Could you check a few things on this model? Use its own coordinates, in mm. A direction names the side the tool comes from. Round coordinates to 2 decimals unless told otherwise and drop trailing zeros. One line per question, with ' | ' between items.
```python
from build123d import *

# Parameters (mm, degrees)
F0_W      = 101.6
F0_H      = 25.4
F1_DEPTH  = 101.6
F1_FACE_W = 101.6
F1_FACE_H = 101.6
F6_DEPTH  = 50.8
F8_DEPTH  = 63.5


with BuildPart() as f1:
    # F0 (on Front) → F1 (new body)
    with BuildSketch(Plane.XZ):
        with Locations((-50.8, -12.7)):
            Rectangle(F0_W, F0_H)
    extrude(amount=F1_DEPTH)

    # F1_face (on face) → F4 section 0
    with BuildSketch(Plane(origin=(-50.8, -50.8, 0), x_dir=(1, 0, 0), z_dir=(0, 0, 1))):
        Rectangle(F1_FACE_W, F1_FACE_H)
    # F3 (on offset) → F4 section 1
    with BuildSketch(Plane.XY.offset(323.85)):
        Polygon((0, -50.8), (-50.8, 0), (-101.6, -50.8), (-50.8, -101.6), align=None)
    loft()

    # F5 (on face) → F6 (cut)
    with BuildSketch(Plane.XY.offset(323.85)):
        with BuildLine():
            ThreePointArc((-46.3098719395, -46.3098719395), (-50.8, -44.45), (-55.2901280605, -46.3098719395))
            Line((-55.2901280605, -46.3098719395), (-50.8, -50.8))
            Line((-50.8, -50.8), (-46.3098719395, -46.3098719395))
        make_face()
        with BuildLine():
            Line((-50.8, -50.8), (-55.2901280605, -46.3098719395))
            ThreePointArc((-55.2901280605, -46.3098719395), (-57.15, -50.8), (-55.2901280605, -55.2901280605))
            Line((-55.2901280605, -55.2901280605), (-50.8, -50.8))
        make_face()
        with BuildLine():
            Line((-46.3098719395, -55.2901280605), (-50.8, -50.8))
            Line((-50.8, -50.8), (-55.2901280605, -55.2901280605))
            ThreePointArc((-55.2901280605, -55.2901280605), (-50.8, -57.15), (-46.3098719395, -55.2901280605))
        make_face()
        with BuildLine():
            Line((-46.3098719395, -46.3098719395), (-50.8, -50.8))
            Line((-50.8, -50.8), (-46.3098719395, -55.2901280605))
            ThreePointArc((-46.3098719395, -55.2901280605), (-44.9333649686, -53.2300397955), (-44.45, -50.8))
            ThreePointArc((-44.45, -50.8), (-44.9333649686, -48.3699602045), (-46.3098719395, -46.3098719395))
        make_face()
    extrude(amount=-F6_DEPTH, mode=Mode.SUBTRACT)

    # F7 (on face) → F8 (cut)
    with BuildSketch(Plane(origin=(0, 0, -25.4), x_dir=(1, 0, 0), z_dir=(0, 0, -1))):
        with BuildLine():
            ThreePointArc((-41.275, 50.8), (-44.0648079092, 57.5351920908), (-50.8, 60.325))
            Line((-50.8, 60.325), (-50.8, 41.275))
            ThreePointArc((-50.8, 41.275), (-44.0648079092, 44.0648079092), (-41.275, 50.8))
        make_face()
        with BuildLine():
            Line((-50.8, 41.275), (-50.8, 60.325))
            ThreePointArc((-50.8, 60.325), (-60.325, 50.8), (-50.8, 41.275))
        make_face()
    extrude(amount=-F8_DEPTH, mode=Mode.SUBTRACT)


solid = f1.part
```
1. I need wall thicknesses on probe 1 along Y at (x, z) = (-50, 15); probe 2 along X at (y, z) = (-50, 19); probe 3 along Y at (x, z) = (-50, 20). Which ranges of each line are inside material? Lowest first, please.
From the geometry:
probe 1: y = -100.47 to -60.29, -41.31 to -1.17 | probe 2: x = -100.13 to -60.29, -41.31 to -1.42 | probe 3: y = -100.11 to -60.29, -41.31 to -1.54
2. If we mould it in two halves opening along X, with no side actions, what happens to faces 4 (the face through (-52, -39, 323.85)), 5 (the face through (-51, -51, 38.1)), 6 (the face through (0, -50, -13))? For each: pulls with the +X half, pulls with the -X half, needs draft (parallel to the pull), parting line crosses it, or undercut.
From the geometry:
face 4: needs draft | face 5: undercut | face 6: pulls with the +X half
3. On a 3-axis mill with a long thin cutter (end or side, diameter ignored), from which of +Z, -Z, +X, -X, +Y, -Y can I reach the whole of each face in a straight line? I mean faces 1 (the face through (-51, -51, 273.05)), 2 (the face through (-42, -47.15, 5.91)), 3 (the face through (-52, 0, -13)). Say none if no direction works.
From the geometry:
face 1: +Z | face 2: -Z | face 3: +Z, -Z, +X, -X, +Y
4. I'm going to push flat-ended pins straight in: pin 1 (6.5 mm diameter, centred on x = -51.5, y = -52, fed in from +Z); pin 2 (1 mm diameter, centred on x = -91, z = 258.5, fed in from +Y); pin 3 (5.5 mm diameter, centred on x = -54, y = -52.5, fed in from -Z). Where does each tip first touch, or does it pass through?
From the geometry:
pin 1: stops at z = 273.05 | pin 2: stops at y = -44.34 | pin 3: stops at z = 38.1
